Part model, mm, in its own coordinate system. A direction names the side the tool comes from. Round coordinates to 2 decimals unless told otherwise and drop trailing zeros. Loops run counter-clockwise (first coordinate to the right, second up) from the corner with the lowest first, then second, coordinate; pieces in that order, holes last. Notation, with made-up numbers: (32, 88.5) -> (48, 88.5) arc R26 cw to (48, 122.5) -> close; hole circle Ø8 at (27.5, 13.25). An arc over 180 degrees is marked (long way). Use a Markdown table: item, result. Add a question column.
Item 1: Probe line 1 (X direction, y = -11.5, z = 9); line 2 (Z direction, x = -49, y = -10); line 3 (Z direction, x = -32.5, y = -2.25). List the from-to ranges inside material, lowest first. Write a range as [from, to].
Item 2: Cut at A-A, the plane x = -48. List the corners of the cut face in (y, z).
Item 3: Which spindle directions (+Z, -Z, +X, -X, +Y, -Y) get a long thin tool onto all of the face, cutting with end or side? Do faces 5 (the face through (-55.5, -7, -1)), 6 (the face through (-1, -6, 103)). Say none if no direction does.
Item 4: Flat gauge pins, fed straight in: pin 1 (2 mm diameter, centred on y = -1.5, z = 80, fed in from +X); pin 2 (2.5 mm diameter, centred on y = -1, z = 45, fed in from -X); pin 3 (14 mm diameter, centred on x = -49, z = -34, fed in from +Y). Where does each tip first touch, or does it go through?
Item 5: Two-plate mould, pull along X, no slides. Class faces 1 (the face through (-67.5, -7, -1)), 2 (the face through (67.5, -7, -1)), 3 (the face through (-1, -6, -103)), 4 (the face through (-57, -3, -7)): pulls with the +X half, pulls with the -X half, needs draft (parallel to the pull), parting line crosses it, or undercut.
Item 6: Cut at C-C, the plane y = -5. List the corners of the cut face in (x, z).
Item 7: Cut at B-B, the plane z = -22.5. List the corners of the cut face in (x, y).
```python
from build123d import *

# Parameters (mm, degrees)
F0_W     = 135
F0_H     = 206
F1_DEPTH = 12
F2_DEPTH = 3
F3_R     = 3


with BuildPart() as f1:
    # F0 (on Front) → F1 (new body)
    with BuildSketch(Plane.XZ):
        Rectangle(F0_W, F0_H)
        with BuildLine():
            ThreePointArc((-17.2, 99), (-16.492893, 98.707107), (-16.2, 98))
            Line((-16.2, 98), (-16.2, -98))
            ThreePointArc((-16.2, -98), (-16.492893, -98.707107), (-17.2, -99))
            Line((-17.2, -99), (-62.2, -99))
            ThreePointArc((-62.2, -99), (-62.907107, -98.707107), (-63.2, -98))
            Line((-63.2, -98), (-63.2, 98))
            ThreePointArc((-63.2, 98), (-62.907107, 98.707107), (-62.2, 99))
            Line((-62.2, 99), (-17.2, 99))
        make_face(mode=Mode.SUBTRACT)
        with BuildLine():
            Line((-16.2, -98), (-16.2, 98))
            ThreePointArc((-16.2, 98), (-16.492893, 98.707107), (-17.2, 99))
            Line((-17.2, 99), (-62.2, 99))
            ThreePointArc((-62.2, 99), (-62.907107, 98.707107), (-63.2, 98))
            Line((-63.2, 98), (-63.2, -98))
            ThreePointArc((-63.2, -98), (-62.907107, -98.707107), (-62.2, -99))
            Line((-62.2, -99), (-17.2, -99))
            ThreePointArc((-17.2, -99), (-16.492893, -98.707107), (-16.2, -98))
        make_face()
        with BuildLine():
            ThreePointArc((-55.5, 91), (-55.207107, 91.707107), (-54.5, 92))
            Line((-54.5, 92), (-24.5, 92))
            ThreePointArc((-24.5, 92), (-23.792893, 91.707107), (-23.5, 91))
            Line((-23.5, 91), (-23.5, -91))
            ThreePointArc((-23.5, -91), (-23.792893, -91.707107), (-24.5, -92))
            Line((-24.5, -92), (-54.5, -92))
            ThreePointArc((-54.5, -92), (-55.207107, -91.707107), (-55.5, -91))
            Line((-55.5, -91), (-55.5, 91))
        make_face(mode=Mode.SUBTRACT)
    extrude(amount=F1_DEPTH)

    # F0 (on Front) → F2 (cut)
    with BuildSketch(Plane.XZ):
        with BuildLine():
            Line((-16.2, -98), (-16.2, 98))
            ThreePointArc((-16.2, 98), (-16.492893, 98.707107), (-17.2, 99))
            Line((-17.2, 99), (-62.2, 99))
            ThreePointArc((-62.2, 99), (-62.907107, 98.707107), (-63.2, 98))
            Line((-63.2, 98), (-63.2, -98))
            ThreePointArc((-63.2, -98), (-62.907107, -98.707107), (-62.2, -99))
            Line((-62.2, -99), (-17.2, -99))
            ThreePointArc((-17.2, -99), (-16.492893, -98.707107), (-16.2, -98))
        make_face()
        with BuildLine():
            ThreePointArc((-55.5, 91), (-55.207107, 91.707107), (-54.5, 92))
            Line((-54.5, 92), (-24.5, 92))
            ThreePointArc((-24.5, 92), (-23.792893, 91.707107), (-23.5, 91))
            Line((-23.5, 91), (-23.5, -91))
            ThreePointArc((-23.5, -91), (-23.792893, -91.707107), (-24.5, -92))
            Line((-24.5, -92), (-54.5, -92))
            ThreePointArc((-54.5, -92), (-55.207107, -91.707107), (-55.5, -91))
            Line((-55.5, -91), (-55.5, 91))
        make_face(mode=Mode.SUBTRACT)
    extrude(amount=F2_DEPTH, mode=Mode.SUBTRACT)

    # F3
    f3_edges = [f1.edges().sort_by_distance(p)[0] for p in [
        (67.5, 0, 0),
        (-67.5, 0, 0),
    ]]
    fillet(f3_edges, radius=F3_R)


solid = f1.part
```
A:
| question | item | result |
|---|---|---|
| 1 | line 1 | x = [-67.5, -55.5], [-23.5, 67.5] |
| 1 | line 2 | z = [-103, -92], [92, 103] |
| 1 | line 3 | z = [-103, -99], [99, 103] |
| 2 | outline | (-12, -103) -> (0, -103) -> (0, -99) -> (-3, -99) -> (-3, -92) -> (-12, -92) -> close; (-12, 92) -> (-3, 92) -> (-3, 99) -> (0, 99) -> (0, 103) -> (-12, 103) -> close |
| 3 | face 5 | +Y, -Y |
| 3 | face 6 | +Z, +X, -X, +Y, -Y |
| 4 | pin 1 | stops at x = 67.46 |
| 4 | pin 2 | stops at x = -67.4 |
| 4 | pin 3 | stops at y = -3 |
| 5 | face 1 | pulls with the -X half |
| 5 | face 2 | pulls with the +X half |
| 5 | face 3 | needs draft |
| 5 | face 4 | undercut |
| 6 | outline | (-67.5, -103) -> (67.5, -103) -> (67.5, 103) -> (-67.5, 103) -> close; hole (-55.5, -91) arc R1 ccw to (-54.5, -92) -> (-24.5, -92) arc R1 ccw to (-23.5, -91) -> (-23.5, 91) arc R1 ccw to (-24.5, 92) -> (-54.5, 92) arc R1 ccw to (-55.5, 91) -> close |
| 7 | outline | (-67.5, -12) -> (-55.5, -12) -> (-55.5, -3) -> (-63.2, -3) -> (-63.2, 0) -> (-64.5, 0) arc R3 ccw to (-67.5, -3) -> close; (-23.5, -12) -> (67.5, -12) -> (67.5, -3) arc R3 ccw to (64.5, 0) -> (-16.2, 0) -> (-16.2, -3) -> (-23.5, -3) -> close |
